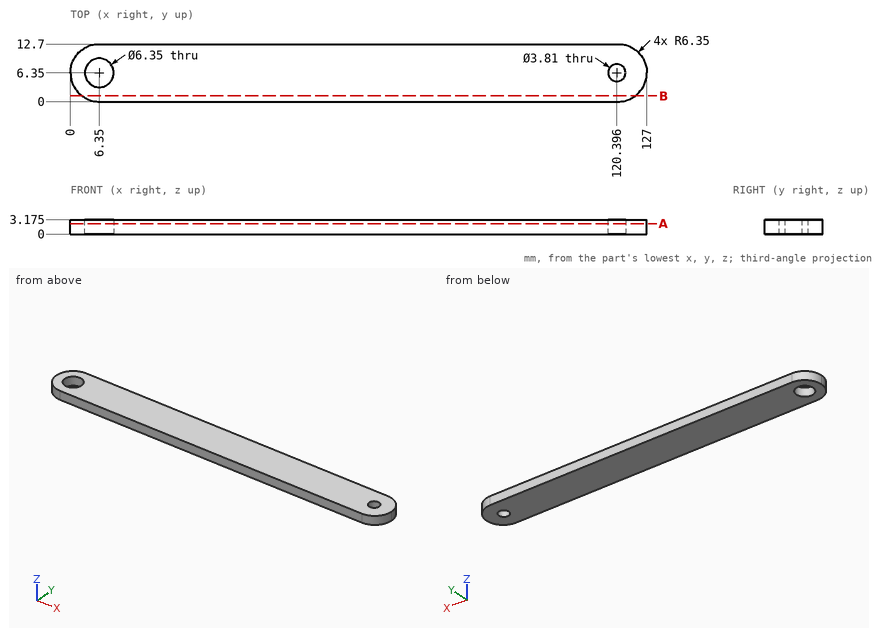
Here's the drawing with two shaded views (mm, measured from the low corner). I have some questions. Round coordinates to 2 decimals unless told otherwise and drop trailing zeros. Loops run counter-clockwise (first coordinate to the right, second up) from the corner with the lowest first, then second, coordinate; pieces in that order, holes last.
1. Suppose I cut it at B-B, the plane y = 1.25. Please give me the cut outline in (x, z) (3 decimals), and give its area (3 significant figures).
Answers:
outline: (2.567, 0) - (124.433, 0) - (124.433, 3.175) - (2.567, 3.175) - close
area: 387 mm2
2. Suppose I cut it at A-A, the plane z = 2.3. Give the number of separate pieces and of enclosed holes in the cut face, and give its area (3 significant figures).
Answers:
separate pieces: 1
enclosed holes: 2
area: 1,540 mm2
3. If I drill on probe 1 along X at (y, z) = (5.25, 0.2); probe 2 along X at (y, z) = (8.75, 1); probe 3 along X at (y, z) = (6, 1.5), over which ranges is the centre line in solid material (lowest first)?
Answers:
probe 1: x = 0.1 to 3.37, 9.33 to 118.84, 121.95 to 126.9
probe 2: x = 0.47 to 4.27, 8.43 to 126.53
probe 3: x = 0.01 to 3.19, 9.51 to 118.52, 122.27 to 126.99
